Source: CAD feature listing. Evaluate the final solid. Frame: model axes, mm. Give positions to 0.01 mm unless a question says otherwise; leave off trailing zeros. Order: outer loops, then holes, each group sorted by start corner. A loop starts at its lowest first (then second) coordinate and runs counter-clockwise, first axis right, second up. Notation, with made-up numbers: M -27,71 L 17,71 A24 cw 17,107 Z; hole C -39.75,-37 d11. An arc over 180 degrees is marked long. Return JSON: item names as keys, results as strings.
from build123d import *

# Parameters (mm, degrees)
CHAMFER_1_SIZE = 1


with BuildPart() as part:
    # 草图1 → 旋转1 (revolve)
    with BuildSketch(Plane(origin=(0, 0, 0), x_dir=(0, 0, -1), z_dir=(1, 0, 0)), mode=Mode.PRIVATE) as revolve_1_sk:
        Polygon((14.3, 83), (-14.3, 83), (-16.5, 87.412517358), (-16.5, 112.5), (16.5, 112.5), (16.5, 87.412517358), align=None)
    revolve(revolve_1_sk.sketch.rotate(Axis((0, 0, 15.038452749), (0, 0, -1)), 90), axis=Axis((0, 0, 15.038452749), (0, 0, -1)))

    # 倒角1
    chamfer_1_edges = [part.edges().sort_by_distance(p)[0] for p in [
        (-112.5, 0, -16.5),
        (-112.5, 0, 16.5),
    ]]
    chamfer(chamfer_1_edges, length=CHAMFER_1_SIZE)


solid = part.part
1. Draft query along Y for faces 1 (the face through (79.167, -24.931, 0.2)), 2 (the face through (79.372, -24.995, -14.407)), 3 (the face through (107.305, -33.792, -0.217)), 4 (the face through (-67, 57, -16.5)). Return one class per face: pulls with the +Y half, pulls with the -Y half, needs draft (parallel to the pull), parting line crosses it, or undercut.
Evaluation:
{"face 1": "undercut", "face 2": "undercut", "face 3": "parting line crosses it", "face 4": "needs draft"}
2. First-contact query: pin 1 (1 mm diameter, centred on x = 62.5, z = -3, fed in from +Y); pin 2 (2 mm diameter, centred on x = 84, z = 11, fed in from -Y); pin 3 (6 mm diameter, centred on y = -78.5, z = 6, fed in from -X). Flat tips, straight axial feed; report the tip coordinate or a pass-through.
Evaluation:
{"pin 1": "stops at y = 93.87", "pin 2": "stops at y = -75.94", "pin 3": "stops at x = -83.4"}
3. Section query A-A (x = 0). Return loops of the section in (y, z), then the cut area to 3 significant figures.
Evaluation:
{"outline": "M -112.5,-15.5 L -111.5,-16.5 L -87.41,-16.5 L -83,-14.3 L -83,14.3 L -87.41,16.5 L -111.5,16.5 L -112.5,15.5 Z; M 83,-14.3 L 87.41,-16.5 L 111.5,-16.5 L 112.5,-15.5 L 112.5,15.5 L 111.5,16.5 L 87.41,16.5 L 83,14.3 Z", "area": "1,930 mm^2"}
4. Section query C-C (z = -11.5). Return loops of the section in (x, y).
Evaluation:
{"outline": "C 0,0 d225; hole C 0,0 d166"}
5. Ray query, probe 1 along Y at (x, z) = (0, 0.5); probe 2 along Y at (x, z) = (10, 4.5); probe 3 along X at (y, z) = (62.5, -9). Return the intervals inside material, ascending.
Evaluation:
{"probe 1": "y = -112.5 to -83, 83 to 112.5", "probe 2": "y = -112.05 to -82.4, 82.4 to 112.05", "probe 3": "x = -93.54 to -54.61, 54.61 to 93.54"}
